Read the model definition and answer for the solid it produces. Units are mm, in the model's axes. Give positions to 0.01 mm unless a question says otherwise; leave off trailing zeros. Order: outer loops, then holes, each group sorted by start corner. A loop starts at its lowest first (then second) coordinate and runs counter-clockwise, first axis right, second up.
Item 1: Given pin 1 Ø15.5 at (y, z) = (-11, 13.5) entering from +X; pin 2 Ø9.5 at (y, z) = (-12, 22) entering from -X, each flat-ended and moving along its own axis, determine where each tip first touches the part or whether it passes through.
Item 2: Find the intervals of material crossed by line 1 along X through (y, z) = (-5.5, 16); line 2 along Y through (x, z) = (48.5, 33.5); line 3 along Y through (x, z) = (71.5, 29.5), in increasing order.
Item 3: A cutting plane is placed at A-A (y = -8.5). Write down the section's boundary in (x, z), plus the area to 3 significant figures.
Item 4: A cutting plane is placed at B-B (z = 10). Write down the section's boundary in (x, y), plus the area to 3 significant figures.
from build123d import *

# Parameters (mm, degrees)
SKETCH1_W           = 125
SKETCH1_H           = 65
BOSS_EXTRUDE1_DEPTH = 35
FILLET1_R           = 2
SKETCH2_W           = 7
SKETCH2_H           = 8.5
BOSS_EXTRUDE2_DEPTH = 15
BOSS_EXTRUDE2_TAPER = 4
SKETCH3_W           = 6.425912995
SKETCH3_H           = 8.003375871
BOSS_EXTRUDE3_DEPTH = 15
BOSS_EXTRUDE3_TAPER = 4


with BuildPart() as part:
    # Sketch1 → Boss-Extrude1 (new body)
    with BuildSketch(Plane.XY):
        Rectangle(SKETCH1_W, SKETCH1_H)
    extrude(amount=BOSS_EXTRUDE1_DEPTH)

    # Fillet1
    fillet1_edges = [part.edges().sort_by_distance(p)[0] for p in [
        (-62.5, 0, 35),
        (0, -32.5, 35),
        (62.5, 0, 35),
        (0, -32.5, 0),
        (-62.5, 0, 0),
        (0, 32.5, 0),
        (62.5, 0, 0),
        (0, 32.5, 35),
        (62.5, -32.5, 17.5),
        (-62.5, -32.5, 17.5),
        (-62.5, 32.5, 17.5),
        (62.5, 32.5, 17.5),
    ]]
    fillet(fillet1_edges, radius=FILLET1_R)

    # Sketch2 → Boss-Extrude2 (add)
    with BuildSketch(Plane(origin=(62.5, 0, 0), x_dir=(0, 0, -1), z_dir=(1, 0, 0))):
        with Locations((-27.977253616, 23.429314173)):
            Rectangle(SKETCH2_W, SKETCH2_H)
    extrude(amount=BOSS_EXTRUDE2_DEPTH, taper=BOSS_EXTRUDE2_TAPER)

    # Sketch3 → Boss-Extrude3 (add)
    with BuildSketch(Plane.ZY.offset(62.5)):
        with Locations((28.744757, -24.829951406)):
            Rectangle(SKETCH3_W, SKETCH3_H)
    extrude(amount=BOSS_EXTRUDE3_DEPTH, taper=BOSS_EXTRUDE3_TAPER)


solid = part.part
Response values:
1. pin 1: stops at x = 62.5
1. pin 2: stops at x = -62.5
2. line 1: x = -62.5 to 62.5
2. line 2: y = -32.44 to 32.44
2. line 3: y = 19.81 to 27.05
3. outline: (-62.5, 2) arc R2 ccw to (-60.5, 0) - (60.5, 0) arc R2 ccw to (62.5, 2) - (62.5, 33) arc R2 ccw to (60.5, 35) - (-60.5, 35) arc R2 ccw to (-62.5, 33) - close
3. area: 4,370 mm2
4. outline: (-62.5, -30.5) arc R2 ccw to (-60.5, -32.5) - (60.5, -32.5) arc R2 ccw to (62.5, -30.5) - (62.5, 30.5) arc R2 ccw to (60.5, 32.5) - (-60.5, 32.5) arc R2 ccw to (-62.5, 30.5) - close
4. area: 8,120 mm2
